```python
from build123d import *

# Parameters (mm, degrees)
SKETCH_R     = 1.6
PAD_DEPTH    = 18
SKETCH001_R  = 1.65
PAD001_DEPTH = 7


with BuildPart() as part:
    # Sketch → Pad (new body)
    with BuildSketch(Plane.XY):
        with BuildLine():
            ThreePointArc((-7.5, 4.25), (-8.207107, 3.957107), (-8.5, 3.25))
            Line((-8.5, -3.25), (-8.5, 3.25))
            ThreePointArc((-8.5, -3.25), (-8.207107, -3.957107), (-7.5, -4.25))
            Line((3.506737, -4.25), (-7.5, -4.25))
            ThreePointArc((3.506737, -4.25), (4.171612, -3.996955), (4.5, -3.365883))
            Line((4.5, 0), (4.5, -3.365883))
            Line((4.5, 0), (6.5, 0))
            Line((6.5, -3.25), (6.5, 0))
            ThreePointArc((6.5, -3.25), (6.792893, -3.957107), (7.5, -4.25))
            Line((11.5, -4.25), (7.5, -4.25))
            ThreePointArc((11.5, -4.25), (12.207107, -3.957107), (12.5, -3.25))
            Line((12.5, 3.25), (12.5, -3.25))
            ThreePointArc((12.5, 3.25), (12.207107, 3.957107), (11.5, 4.25))
            Line((7.5, 4.25), (11.5, 4.25))
            ThreePointArc((7.5, 4.25), (6.793016, 3.957229), (6.5, 3.250346))
            Line((6.5, 0.001), (6.5, 3.250346))
            Line((4.5, 0.001), (6.5, 0.001))
            Line((4.5, 3.25), (4.5, 0.001))
            ThreePointArc((4.5, 3.25), (4.207107, 3.957107), (3.5, 4.25))
            Line((-7.5, 4.25), (3.5, 4.25))
        make_face()
        Circle(SKETCH_R, mode=Mode.SUBTRACT)
    extrude(amount=PAD_DEPTH)

    # Sketch001 → Pad001 (join)
    with BuildSketch(Plane.XY):
        with BuildLine():
            ThreePointArc((-8, 4.5), (-8.707107, 4.207107), (-9, 3.5))
            Line((-9, -3.5), (-9, 3.5))
            ThreePointArc((-9, -3.5), (-8.707107, -4.207107), (-8, -4.5))
            Line((24, -4.5), (-8, -4.5))
            ThreePointArc((24, -4.5), (24.707107, -4.207107), (25, -3.5))
            Line((25, 3.5), (25, -3.5))
            ThreePointArc((25, 3.5), (24.707107, 4.207107), (24, 4.5))
            Line((-8, 4.5), (24, 4.5))
        make_face()
        Circle(SKETCH001_R, mode=Mode.SUBTRACT)
    extrude(amount=-PAD001_DEPTH)


solid = part.part
```
Here's how the part is built. I have some questions about the finished solid (model axes, mm). A direction names the side the tool comes from. Give positions to 0.01 mm unless a question says otherwise; leave off trailing zeros. Order: outer loops, then holes, each group sorted by start corner. A loop starts at its lowest first (then second) coordinate and runs counter-clockwise, first axis right, second up. Notation, with made-up numbers: (18.25, -7.75) -> (38.25, -7.75) arc R26 cw to (38.25, 29.25) -> close; hole circle Ø1 at (-15.5, 57.5). An arc over 180 degrees is marked (long way). Use CSV: the item, a comma, the result in double quotes. Start each with the question number.
Item 1: Thinking about a two-plate mould opening in X: for faces 5 (the cylindrical face through (6.801, 3.965, 8.874)), 6 (the cylindrical face through (-8.715, -4.199, -3.451)), 7 (the flat face through (8, -4.5, -3)), 8 (the cylindrical face through (24.715, 4.199, -3.451)), which applies, pulls with the +X half, pulls with the -X half, needs draft (parallel to the pull), parting line crosses it, or undercut?
Item 2: If I drill on probe 1 along Y at (x, z) = (0, -2.5); probe 2 along X at (y, z) = (3, 12.5); probe 3 along Y at (x, z) = (0, 5.75), over which ranges is the centre line in solid material (lowest first)? Write a range as [from, to].
Item 3: Suppose I cut it at A-A (x = 0). List the corners of the cut face in (y, z) for me.
Item 4: Suppose I cut it at C-C (z = 12.75). List the corners of the cut face in (x, y) for me.
Item 5: Suppose I cut it at D-D (y = -0.5). List the corners of the cut face in (x, z) for me, and give its area (3 significant figures).
Item 6: I'm going to push flat-ended pins straight in: P1, Ø12, axis at x = 19, z = 10.5, coming from the -Y side; P2, Ø2.5, axis at x = 0, y = -0.5, coming from the -Z side; P3, Ø2.5, axis at y = -1.5, z = 6, coming from the -X side; P4, Ø1.6, axis at x = 5.5, z = 12, coming from the +Y side. Where does each tip first touch, or does it pass through?
Item 7: On a 3-axis mill with a long thin cutter (end or side, diameter ignored), from which of +Z, -Z, +X, -X, +Y, -Y can I reach the whole of each face in a straight line? I mean faces 1 (the flat face through (9, 4.25, 9)), 2 (the flat face through (6.5, -2, 9)), 3 (the cylindrical face through (-1.216, 1.115, -3.451)), 4 (the flat face through (-2, -4.25, 9)). Say none if no direction works.
Item 8: Suppose I cut it at B-B (y = 2.75). List the corners of the cut face in (x, z) for me.
Answer block:
1,face 5,"undercut"
1,face 6,"pulls with the -X half"
1,face 7,"needs draft"
1,face 8,"pulls with the +X half"
2,probe 1,"y = [-4.5, -1.65], [1.65, 4.5]"
2,probe 2,"x = [-8.5, 4.5], [6.5, 12.5]"
2,probe 3,"y = [-4.25, -1.6], [1.6, 4.25]"
3,outline,"(-4.5, -7) -> (-1.65, -7) -> (-1.65, 0) -> (-1.6, 0) -> (-1.6, 18) -> (-4.25, 18) -> (-4.25, 0) -> (-4.5, 0) -> close; (1.6, 0) -> (1.65, 0) -> (1.65, -7) -> (4.5, -7) -> (4.5, 0) -> (4.25, 0) -> (4.25, 18) -> (1.6, 18) -> close"
4,outline,"(-8.5, -3.25) arc R1 ccw to (-7.5, -4.25) -> (3.51, -4.25) arc R1 ccw to (4.5, -3.37) -> (4.5, 0) -> (6.5, 0) -> (6.5, -3.25) arc R1 ccw to (7.5, -4.25) -> (11.5, -4.25) arc R1 ccw to (12.5, -3.25) -> (12.5, 3.25) arc R1 ccw to (11.5, 4.25) -> (7.5, 4.25) arc R1 ccw to (6.5, 3.25) -> (6.5, 0) -> (4.5, 0) -> (4.5, 3.25) arc R1 ccw to (3.5, 4.25) -> (-7.5, 4.25) arc R1 ccw to (-8.5, 3.25) -> close; hole circle Ø3.2 at (0, 0)"
5,outline,"(-9, -7) -> (-1.57, -7) -> (-1.57, 0) -> (-1.52, 0) -> (-1.52, 18) -> (-8.5, 18) -> (-8.5, 0) -> (-9, 0) -> close; (1.52, 0) -> (1.57, 0) -> (1.57, -7) -> (25, -7) -> (25, 0) -> (12.5, 0) -> (12.5, 18) -> (6.5, 18) -> (6.5, 0) -> (4.5, 0) -> (4.5, 18) -> (1.52, 18) -> close"
5,area,"503 mm^2"
6,P1,"passes through"
6,P2,"stops at z = -7"
6,P3,"stops at x = -8.5"
6,P4,"stops at y = 0"
7,face 1,"+Z, +X, -X, +Y"
7,face 2,"+Z, -Y"
7,face 3,"-Z"
7,face 4,"+Z, +X, -X, -Y"
8,outline,"(-9, -7) -> (25, -7) -> (25, 0) -> (12.5, 0) -> (12.5, 18) -> (6.5, 18) -> (6.5, 0) -> (4.5, 0) -> (4.5, 18) -> (-8.5, 18) -> (-8.5, 0) -> (-9, 0) -> close"
